Part print with two shaded views. Sizes in mm from the minimum x, y, z corner. A direction names the side the tool comes from. Round coordinates to 2 decimals unless told otherwise and drop trailing zeros. Loops run counter-clockwise (first coordinate to the right, second up) from the corner with the lowest first, then second, coordinate; pieces in that order, holes last. Notation, with made-up numbers: M 45.25,41 L 60.25,41 A7 ccw 60.25,46 Z; hole C 5,6 d9. An arc over 180 degrees is marked long. Answer as CSV lines item,"result". Start each with the question number.
Item 1: Band-saw the part on B-B (y = 3). Give the cut face in (x, z).
Item 2: Mould opens along Z. For the marked faces 1, 2 and 3 say: pulls with the +Z half, pulls with the -Z half, needs draft (parallel to the pull), parting line crosses it, or undercut.
Item 3: Wall check: line 1 (Y direction, x = 4.75, z = 10.5); line 2 (Y direction, x = 7, z = 8.25); line 3 (X direction, y = 15.25, z = 5.25). Give the ranges that are in metal, low to high.
Item 4: Band-saw the part on A-A (z = 6.5). Give the cut face in (x, y).
Item 5: Drop flat-ended pins along their axis: pin 1 Ø1 at (y, z) = (12, 9.5) entering from +X; pin 2 Ø6 at (x, y) = (5, 14.5) entering from -Z; pin 3 Ø4 at (y, z) = (21, 10) entering from -X (1 decimal). Give the stop position or say it passes through.
Item 6: Which spindle directions (+Z, -Z, +X, -X, +Y, -Y) get a long thin tool onto all of the face, cutting with end or side? Do the marked faces 4, 5 and 6. Say none if no direction does.
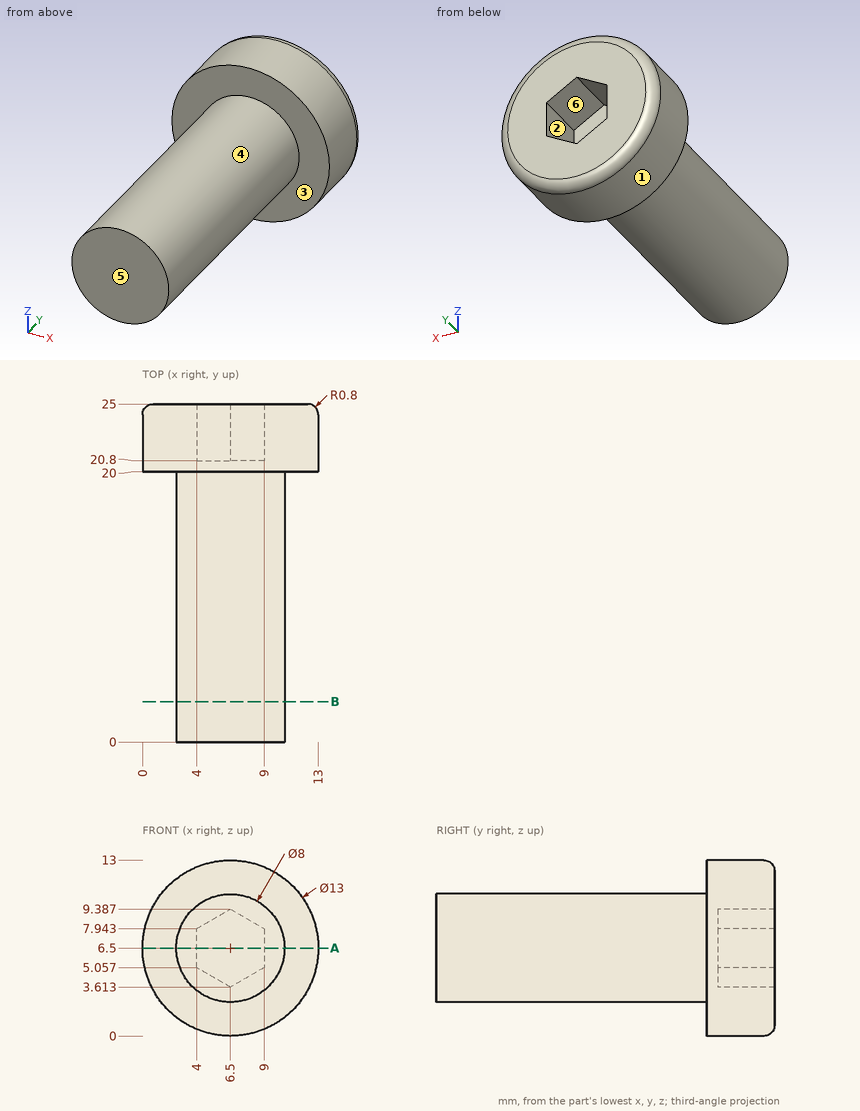
Answer block:
1,outline,"C 6.5,6.5 d8"
2,face 1,"parting line crosses it"
2,face 2,"undercut"
2,face 3,"needs draft"
3,line 1,"y = 20 to 25"
3,line 2,"y = 0 to 20.8"
3,line 3,"x = 2.7 to 10.3"
4,outline,"M 0,20 L 2.5,20 L 2.5,0 L 10.5,0 L 10.5,20 L 13,20 L 13,24.2 A0.8 ccw 12.2,25 L 9,25 L 9,20.8 L 4,20.8 L 4,25 L 0.8,25 A0.8 ccw 0,24.2 Z"
5,pin 1,"stops at x = 9.62"
5,pin 2,"stops at z = 2.5"
5,pin 3,"stops at x = 0.2"
6,face 4,"-Y"
6,face 5,"+Z, -Z, +X, -X, -Y"
6,face 6,"+Y"
